Input: part model. Units: mm. Frame: model coordinates. A direction names the side the tool comes from. Give positions to 0.01 mm unless a question says otherwise; leave off trailing zeros. Loops run counter-clockwise (first coordinate to the right, second up) from the corner with the lowest first, then second, coordinate; pieces in that order, holes last. Notation, with made-up numbers: (8.5, -8.75) -> (29.5, -8.75) arc R14 cw to (29.5, -2.75) -> close; hole circle Ø11 at (6.25, 12). An arc over 180 degrees is marked (long way). Use CSV: the item, a comma, the result in double quotes.
```python
from build123d import *

# Parameters (mm, degrees)
SKETCH1_R           = 7
SKETCH1_R_2         = 2.05
BOSS_EXTRUDE1_DEPTH = 2


with BuildPart() as part:
    # Sketch1 → Boss-Extrude1 (new body)
    with BuildSketch(Plane(origin=(0, 0, 0), x_dir=(1, 0, 0), z_dir=(0, 1, 0))):
        with BuildLine():
            Line((-8.880747298, 1.460249099), (-13.946998799, -29.3510004))
            ThreePointArc((-13.946998799, -29.3510004), (-13.049262075, -32.588822281), (-10, -34))
            Line((-10, -34), (10, -34))
            ThreePointArc((10, -34), (13.049262075, -32.588822281), (13.946998799, -29.3510004))
            Line((13.946998799, -29.3510004), (8.880747298, 1.460249099))
            ThreePointArc((8.880747298, 1.460249099), (0, 9), (-8.880747298, 1.460249099))
        make_face()
        with Locations(Location((0, 0, 0), (0, 0, 270))):
            Circle(SKETCH1_R, mode=Mode.SUBTRACT)
        with Locations(Location((-10, -30, 0), (0, 0, 270))):
            Circle(SKETCH1_R_2, mode=Mode.SUBTRACT)
        with Locations(Location((10, -30, 0), (0, 0, 90))):
            Circle(SKETCH1_R_2, mode=Mode.SUBTRACT)
        with BuildLine():
            Line((-5.494764199, -8.763992606), (-8.269727852, -25.640394709))
            ThreePointArc((-8.269727852, -25.640394709), (-8.197420113, -26.207361672), (-7.826382522, -26.642115687))
            ThreePointArc((-7.826382522, -26.642115687), (-6.950737925, -27.411177719), (-6.333939444, -28.4))
            ThreePointArc((-6.333939444, -28.4), (-5.965146863, -28.836660027), (-5.417424305, -29))
            Line((-5.417424305, -29), (5.417424305, -29))
            ThreePointArc((5.417424305, -29), (5.965146863, -28.836660027), (6.333939444, -28.4))
            ThreePointArc((6.333939444, -28.4), (6.950737925, -27.411177719), (7.826382522, -26.642115687))
            ThreePointArc((7.826382522, -26.642115687), (8.197420113, -26.207361672), (8.269727852, -25.640394709))
            Line((8.269727852, -25.640394709), (5.494764199, -8.763992606))
            ThreePointArc((5.494764199, -8.763992606), (4.960973443, -8.03471113), (4.057213049, -8.033618256))
            ThreePointArc((4.057213049, -8.033618256), (0, -9), (-4.057213049, -8.033618256))
            ThreePointArc((-4.057213049, -8.033618256), (-4.960973443, -8.03471113), (-5.494764199, -8.763992606))
        make_face(mode=Mode.SUBTRACT)
    extrude(amount=BOSS_EXTRUDE1_DEPTH)


solid = part.part
```
1) Section query C-C (y = 1.05). Return loops of the section in (x, z), then the cut area to 3 significant figures.
From the geometry:
outline,"(-13.95, 29.35) -> (-8.88, -1.46) arc R9 ccw to (8.88, -1.46) -> (13.95, 29.35) arc R4 ccw to (10, 34) -> (-10, 34) arc R4 ccw to start; hole circle Ø4.1 at (-10, 30); hole (-8.27, 25.64) -> (-5.49, 8.76) arc R1 ccw to (-4.06, 8.03) arc R9 cw to (4.06, 8.03) arc R1 ccw to (5.49, 8.76) -> (8.27, 25.64) arc R1 ccw to (7.83, 26.64) arc R4 cw to (6.33, 28.4) arc R1 ccw to (5.42, 29) -> (-5.42, 29) arc R1 ccw to (-6.33, 28.4) arc R4 cw to (-7.83, 26.64) arc R1 ccw to start; hole circle Ø14 at (0, 0); hole circle Ø4.1 at (10, 30)"
area,"464 mm^2"
2) Mould query, pull axis Z, two halves, no side actions, for faces 3 (the cylindrical face through (0, 1, -9)), 4 (the cylindrical face through (8.2, 1, 26.2)), 5 (the flat face through (0, 1, 34)). Classes: pulls with the +Z half, pulls with the -Z half, needs draft (parallel to the pull), parting line crosses it, or undercut.
From the geometry:
face 3,"pulls with the -Z half"
face 4,"undercut"
face 5,"pulls with the +Z half"
3) Section query A-A (z = 30). Return loops of the section in (x, y), then the cut area to 3 significant figures.
From the geometry:
outline,"(-14, 0) -> (-12.05, 0) -> (-12.05, 2) -> (-14, 2) -> close; (-7.95, 0) -> (7.95, 0) -> (7.95, 2) -> (-7.95, 2) -> close; (12.05, 0) -> (14, 0) -> (14, 2) -> (12.05, 2) -> close"
area,"39.6 mm^2"
4) Ray query, line 1 (X direction, y = 0.5, z = 30); line 2 (Z direction, x = 1.25, y = 0.1); line 3 (Z direction, x = 1.75, y = 0.7). Return the intervals inside material, ascending.
From the geometry:
line 1,"x = -14 to -12.05, -7.95 to 7.95, 12.05 to 14"
line 2,"z = -8.91 to -6.89, 6.89 to 8.91, 29 to 34"
line 3,"z = -8.83 to -6.78, 6.78 to 8.83, 29 to 34"
5) Section query B-B (x = -2.5). Return loops of the section in (y, z), then the cut area to 3 significant figures.
From the geometry:
outline,"(0, -8.65) -> (2, -8.65) -> (2, -6.54) -> (0, -6.54) -> close; (0, 6.54) -> (2, 6.54) -> (2, 8.65) -> (0, 8.65) -> close; (0, 29) -> (2, 29) -> (2, 34) -> (0, 34) -> close"
area,"18.4 mm^2"
6) Section query D-D (z = 6). Return loops of the section in (x, y), then the cut area to 3 significant figures.
From the geometry:
outline,"(-10.11, 0) -> (-3.61, 0) -> (-3.61, 2) -> (-10.11, 2) -> close; (3.61, 0) -> (10.11, 0) -> (10.11, 2) -> (3.61, 2) -> close"
area,"26.0 mm^2"
7) Reachability of faces 1 (the cylindrical face through (-6.96, 0.99, 27.4)), 2 (the flat face through (-6.4, 0, 12.2)) from +Z, -Z, +X, -X, +Y, -Y: full face, straight path, thin tool, end or side. Return the list, or none.
From the geometry:
face 1,"+Y, -Y"
face 2,"+Z, -Z, +X, -X, -Y"
